```python
from build123d import *

# Parameters (mm, degrees)
F0_R      = 16.4973
F1_DEPTH  = 3.999992
F2_R      = 0.79375
F3_R      = 1.5875
F4_DEPTH  = 13.208
F5_R      = 1.5875
F6_DEPTH  = 12.7
F7_R      = 1.5875
F8_DEPTH  = 25.4
F9_R      = 1.5875
F10_DEPTH = 25.4
F11_R     = 1.5875
F12_DEPTH = 25.4
F13_R     = 1.5875
F14_DEPTH = 25.4
F15_R     = 1.5875
F16_DEPTH = 25.4
F17_R     = 1.5875
F18_DEPTH = 25.4
F19_R     = 5.55625
F20_DEPTH = 1.5875
F21_R     = 2.38125
F22_DEPTH = 1.5875
F24_R     = 14.053096
F24_R_2   = 12.049687
F25_DEPTH = 0.396875
F26_R     = 3.175
F27_DEPTH = 7.9375
F29_R     = 1.5875
F30_DEPTH = 7.9375


with BuildPart() as f1:
    # F0 (on Front) → F1 (new body)
    with BuildSketch(Plane.XZ):
        with Locations((-21.238506, 19.895638)):
            Circle(F0_R)
    extrude(amount=-F1_DEPTH)

    # F2
    f2_edges = [f1.edges().sort_by_distance(p)[0] for p in [
        (-37.735806, 0, 19.895638),
        (-37.735806, 3.999992, 19.895638),
    ]]
    fillet(f2_edges, radius=F2_R)

    # F3 (on face) → F4 (cut)
    with BuildSketch(Plane.XZ):
        with Locations((-21.463407, 28.544784)):
            Circle(F3_R)
    extrude(amount=-F4_DEPTH, mode=Mode.SUBTRACT)

    # F5 (on face) → F6 (cut)
    with BuildSketch(Plane.XZ):
        with Locations((-21.240363, 11.091588)):
            Circle(F5_R)
    extrude(amount=-F6_DEPTH, mode=Mode.SUBTRACT)

    # F7 (on face) → F8 (cut)
    with BuildSketch(Plane.XZ):
        with Locations((-29.88332, 19.734545)):
            Circle(F7_R)
    extrude(amount=-F8_DEPTH, mode=Mode.SUBTRACT)

    # F9 (on face) → F10 (cut)
    with BuildSketch(Plane.XZ):
        with Locations((-12.26284, 19.957587)):
            Circle(F9_R)
    extrude(amount=-F10_DEPTH, mode=Mode.SUBTRACT)

    # F11 (on face) → F12 (cut)
    with BuildSketch(Plane.XZ):
        with Locations((-27.7644, 25.645211)):
            Circle(F11_R)
    extrude(amount=-F12_DEPTH, mode=Mode.SUBTRACT)

    # F13 (on face) → F14 (cut)
    with BuildSketch(Plane.XZ):
        with Locations((-14.772085, 25.868254)):
            Circle(F13_R)
    extrude(amount=-F14_DEPTH, mode=Mode.SUBTRACT)

    # F15 (on face) → F16 (cut)
    with BuildSketch(Plane.XZ):
        with Locations((-27.708638, 13.823877)):
            Circle(F15_R)
    extrude(amount=-F16_DEPTH, mode=Mode.SUBTRACT)

    # F17 (on face) → F18 (cut)
    with BuildSketch(Plane.XZ):
        with Locations((-14.381759, 13.377788)):
            Circle(F17_R)
    extrude(amount=-F18_DEPTH, mode=Mode.SUBTRACT)

    # F19 (on face) → F20 (join)
    with BuildSketch(Plane.XZ):
        with Locations((-21.238506, 19.895638)):
            Circle(F19_R)
    extrude(amount=F20_DEPTH)

    # F21 (on face) → F22 (join)
    with BuildSketch(Plane.XZ.offset(1.5875)):
        with Locations((-21.238506, 19.895638)):
            Circle(F21_R)
    extrude(amount=F22_DEPTH)

    # F24 (on face) → F25 (join)
    with BuildSketch(Plane.XZ):
        with Locations((-21.182381, 19.857397)):
            Circle(F24_R)
        with Locations((-21.238506, 19.895638)):
            Circle(F24_R_2, mode=Mode.SUBTRACT)
    extrude(amount=F25_DEPTH)

    # F26 (on face) → F27 (join)
    with BuildSketch(Plane(origin=(0, 3.999992, 0), x_dir=(-1, 0, 0), z_dir=(0, 1, 0))):
        with Locations((21.238506, 19.895638)):
            Circle(F26_R)
    extrude(amount=F27_DEPTH)

    # F29 (on face) → F30 (cut)
    with BuildSketch(Plane(origin=(0, 11.937492, 0), x_dir=(-1, 0, 0), z_dir=(0, 1, 0))):
        with Locations((21.264283, 19.865673)):
            Circle(F29_R)
    extrude(amount=-F30_DEPTH, mode=Mode.SUBTRACT)


solid = f1.part
```
Part model, mm, in its own coordinate system. A direction names the side the tool comes from. Coordinates: 2 decimals unless noted, no trailing zeros.
Item 1: Slice it at A-A (y = 1.5). Count the separate pieces of the cut face and the enclosed holes in it, and give its area (3 significant figures).
Item 2: Mould opens along X. For faces 4 (the face through (-12.37, 1.983, 33.806)), 5 (the face through (-21, 4, 24)), 6 (the face through (-15.12, 1.97, 24.32)) say: released by +X, released by -X, zero draft, split by the parting line, or undercut.
Item 3: Pin check, flat tips, straight feed: pin 1 (4 mm diameter, centred on x = -12.26, z = 19.96, fed in from +Y); pin 2 (3 mm diameter, centred on x = -9, z = 15.5, fed in from -Y); pin 3 (8 mm diameter, centred on y = -1.5, z = 9, fed in from +X); pin 4 (5.5 mm diameter, centred on x = -19, z = 22, fed in from -Y) (3 decimals). Stop position of each tip, or through.
Item 4: Which spindle directions (+Z, -Z, +X, -X, +Y, -Y) get a long thin tool onto all of the face, cutting with end or side? Do faces 1 (the face through (-31.8, 0, 29.3)), 2 (the face through (-21, 4, 20)), 3 (the face through (-29.295, 1.972, 13.894)). Say none if no direction does.
Item 5: Probe line 1 (Z direction, x = -26.5, y = 0.25); line 2 (Y direction, x = -34.5, z = 24); line 3 (Y direction, x = -18, z = 20.5). List the from-to ranges inside material, lowest first.
Results found:
1. separate pieces: 1
1. enclosed holes: 8
1. area: 792 mm2
2. face 4: split by the parting line
2. face 5: zero draft
2. face 6: undercut
3. pin 1: stops at y = 4
3. pin 2: stops at y = -0.4
3. pin 3: stops at x = -6.57
3. pin 4: stops at y = -3.175
4. face 1: -Y
4. face 2: +Y
4. face 3: +Y, -Y
5. line 1: z = 4.49 to 12.79, 14.85 to 24.69, 26.61 to 35.3
5. line 2: y = -0.4 to 4
5. line 3: y = -1.59 to 4
